```python
from build123d import *

# Parameters (mm, degrees)
SKETCH1_W           = 101.6
SKETCH1_H           = 63.5
BOSS_EXTRUDE1_DEPTH = 3.175
CUT_EXTRUDE1_DEPTH  = 120.85362166
CUT_EXTRUDE2_DEPTH  = 120.85362166
SKETCH5_R           = 2.413
CUT_EXTRUDE3_DEPTH  = 120.85362166


with BuildPart() as part:
    # Sketch1 → Boss-Extrude1 (new body)
    with BuildSketch(Plane.XY):
        with Locations((50.8, 31.75)):
            Rectangle(SKETCH1_W, SKETCH1_H)
    extrude(amount=BOSS_EXTRUDE1_DEPTH)

    # Sketch2 → Cut-Extrude1 (cut, through all)
    with BuildSketch(Plane.XY.offset(3.175)):
        Polygon((101.6, 31.209692887), (79.746737775, 0), (101.6, 0), align=None)
        Polygon((101.6, 36.749322221), (66.100651578, 63.5), (101.6, 63.5), align=None)
    extrude(amount=-CUT_EXTRUDE1_DEPTH, mode=Mode.SUBTRACT)

    # Sketch3 → Cut-Extrude2 (cut, through all)
    with BuildSketch(Plane.XY.offset(3.175)):
        Polygon((21.853262225, 63.5), (0, 32.290307113), (0, 63.5), align=None)
        Polygon((0, 0), (0, 26.750677779), (35.499348422, 0), align=None)
    extrude(amount=-CUT_EXTRUDE2_DEPTH, mode=Mode.SUBTRACT)

    # Sketch5 → Cut-Extrude3 (cut, through all)
    with BuildSketch(Plane.XY.offset(3.175)):
        with Locations((47.958119633, 53.403997063)):
            Circle(SKETCH5_R)
        with Locations((51.894556786, 42.802795542)):
            Circle(SKETCH5_R)
        with Locations((59.154907323, 25.360400118)):
            Circle(SKETCH5_R)
        with Locations((65.389464521, 12.10291712)):
            Circle(SKETCH5_R)
        with Locations((56.503056774, 33.600657948)):
            Circle(SKETCH5_R)
    extrude(amount=-CUT_EXTRUDE3_DEPTH, mode=Mode.SUBTRACT)


solid = part.part
```
CAD build for the part. Positions are in the model's coordinates, mm. Coordinates: 2 decimals unless noted, no trailing zeros. Order: outer loops, then holes, each group sorted by start corner. A loop starts at its lowest first (then second) coordinate and runs counter-clockwise, first axis right, second up. Notation, with made-up numbers: (-9.5, 44) - (46.5, 44) arc R18 cw to (46.5, 48) - close; hole circle Ø10 at (-22, -11.75). An arc over 180 degrees is marked (long way). Use a Markdown table: item, result. Add a question column.
(1) Saw through at D-D (x = 76). Give the cut face in (y, z) (3 decimals), then the cut area to 3 significant figures.
(2) Saw through at C-C (y = 19.5). Give the cut face in (x, z) (3 decimals).
(3) Flat gauge pin, fed straight in: pin 1 (3 mm diameter, centred on x = 56.5, y = 33.6, fed in from +Z). Where does the tip first touch, or does it go through?
(4) Saw through at B-B (z = 2.3). Give the cut face in (x, y).
(5) Saw through at A-A (x = 48). Give the cut face in (y, z) (3 decimals), then the cut area to 3 significant figures.
(6) Drill centre lines: line 1 along X through (y, z) = (35, 1); line 2 along X through (y, z) = (43, 1.8); line 3 along Y through (x, z) = (47, 2.6). Where is each one in solid material? Low to high. Write a range as [from, to].
(7) Pull direction X, two halves, no side cores. Call faces 1 (the face through (56.744, 25.466, 1.61)), 2 (the face through (50, 32, 0)), 3 (the face through (101.6, 34, 2)): +X half, -X half, draft (parallel to the pull), parting line (faces both ways), or undercut.
Solved:
| question | item | result |
|---|---|---|
| 1 | outline | (0, 0) - (56.04, 0) - (56.04, 3.175) - (0, 3.175) - close |
| 1 | area | 178 mm² |
| 2 | outline | (9.622, 0) - (93.401, 0) - (93.401, 3.175) - (9.622, 3.175) - close |
| 3 | pin 1 | passes through |
| 4 | outline | (0, 26.75) - (35.5, 0) - (79.75, 0) - (101.6, 31.21) - (101.6, 36.75) - (66.1, 63.5) - (21.85, 63.5) - (0, 32.29) - close; hole circle Ø4.83 at (47.96, 53.4); hole circle Ø4.83 at (51.89, 42.8); hole circle Ø4.83 at (56.5, 33.6); hole circle Ø4.83 at (59.15, 25.36); hole circle Ø4.83 at (65.39, 12.1) |
| 5 | outline | (0, 0) - (50.991, 0) - (50.991, 3.175) - (0, 3.175) - close; (55.817, 0) - (63.5, 0) - (63.5, 3.175) - (55.817, 3.175) - close |
| 5 | area | 186 mm² |
| 6 | line 1 | x = [1.9, 54.54], [58.47, 101.6] |
| 6 | line 2 | x = [7.5, 49.49], [54.3, 93.31] |
| 6 | line 3 | y = [0, 51.19], [55.62, 63.5] |
| 7 | face 1 | undercut |
| 7 | face 2 | draft |
| 7 | face 3 | +X half |
